The listing builds one solid part. Answer for the finished solid, in the listing's coordinates (mm). Give positions to 0.01 mm unless a question says otherwise; leave off trailing zeros. Write each loop counter-clockwise with the first axis right and the second up, starting at its lowest first coordinate (ties: lowest second). Pieces come first, ordered by that corner, then holes. Notation, with made-up numbers: M -2,69 L 46,69 A25 cw 46,97 Z; hole C 31,50.25 d7. An arc over 180 degrees is marked long. Answer as a JSON object with one key per item and string values.
Autodesk Inventor part; units mm, degrees
ref_plane "YZ Plane" through (0, 0, 0) normal (1, 0, 0) x (0, 1, 0)
ref_plane "XZ Plane" through (0, 0, 0) normal (0, 1, 0) x (-1, 0, 0)
ref_plane "XY Plane" through (0, 0, 0) normal (0, 0, 1) x (1, 0, 0)
sketch "スケッチ1" plane through (0, 0, 0) normal (0, 1, 0) x (-1, 0, 0)
  line L0 (15, -15) -> (-15, -15)
  line L1 (-15, -15) -> (-15, 15)
  line L2 (-15, 15) -> (15, 15)
  line L3 (15, 15) -> (15, -15)
  line L4 (15, -15) -> (-15, 15) construction
  line L5 (-15, -15) -> (15, 15) construction
  point P0 (0, 0)
  point P1 (0, 0)
  dimension "d0" = 30
  dimension "d1" = 30
extrude "押し出し1" add sketch "スケッチ1" along normal blind 1.6
sketch "スケッチ3" plane through (0, 1.6, 0) normal (0, 1, 0) x (1, 0, 0)
  point P0 (0, 0)
  point P1 (0, 0)
  dimension "d17" = 0
hole "穴2" at (0, 1.6, 0) direction (0, -1, 0) diameter 8 depth 4.8
sketch "スケッチ4" plane through (0, 1.6, 0) normal (0, 1, 0) x (1, 0, 0)
  line L0 (15, 15) -> (-15, 15)
  line L1 (15, -15) -> (15, 15)
  point P0 (0, 0)
  point P1 (-9, -9)
  point P2 (9, -9)
  point P3 (9, 9)
  point P4 (-9, 9)
  dimension "d27" = 360
  dimension "d36" = 6
  dimension "d37" = 6
hole "穴3" at (-9, 1.6, 9) at (9, 1.6, 9) at (9, 1.6, -9) at (-9, 1.6, -9) direction (0, -1, 0) diameter 3.4036 depth 1.6
properties part number "pcb" material "フェノール樹脂"
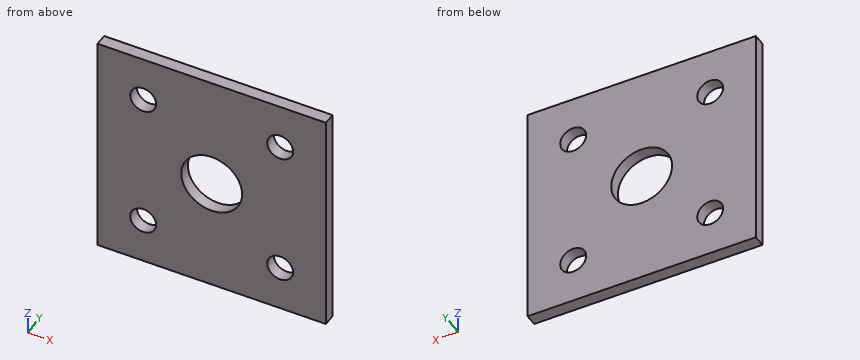
1. A cutting plane is placed at C-C, the plane x = 9. Give the vertices of the cut face in (y, z), plus the area to 3 significant figures.
Verdict:
{"outline": "M 0,-15 L 1.6,-15 L 1.6,-10.7 L 0,-10.7 Z; M 0,-7.3 L 1.6,-7.3 L 1.6,7.3 L 0,7.3 Z; M 0,10.7 L 1.6,10.7 L 1.6,15 L 0,15 Z", "area": "37.1 mm2"}
2. Consider line 1 along X through (y, z) = (0.95, -9); line 2 along Z through (x, y) = (7.75, 0.25). Determine where each line is inside the solid, lowest interval first.
Verdict:
{"line 1": "x = -15 to -10.7, -7.3 to 7.3, 10.7 to 15", "line 2": "z = -15 to -10.15, -7.85 to 7.85, 10.15 to 15"}
3. A cutting plane is placed at A-A, the plane x = 0. Give the vertices of the cut face in (y, z).
Verdict:
{"outline": "M 0,-15 L 1.6,-15 L 1.6,-4 L 0,-4 Z; M 0,4 L 1.6,4 L 1.6,15 L 0,15 Z"}
4. A cutting plane is placed at D-D, the plane z = 0. Give the vertices of the cut face in (x, y).
Verdict:
{"outline": "M -15,0 L -4,0 L -4,1.6 L -15,1.6 Z; M 4,0 L 15,0 L 15,1.6 L 4,1.6 Z"}
5. A cutting plane is placed at B-B, the plane z = 9. Give the vertices of the cut face in (x, y), plus the area to 3 significant figures.
Verdict:
{"outline": "M -15,0 L -10.7,0 L -10.7,1.6 L -15,1.6 Z; M -7.3,0 L 7.3,0 L 7.3,1.6 L -7.3,1.6 Z; M 10.7,0 L 15,0 L 15,1.6 L 10.7,1.6 Z", "area": "37.1 mm2"}
